```python
from build123d import *

# Parameters (mm, degrees)
CORTAR_EXTRUIR1_DEPTH      = 10
CORTAR_EXTRUIR1_DEPTH_BACK = 10
CROQUIS2_W                 = 11.9
CROQUIS2_H                 = 2.7
CORTAR_EXTRUIR2_DEPTH      = 10
CORTAR_EXTRUIR2_DEPTH_BACK = 10
CROQUIS4_W                 = 1
CROQUIS4_H                 = 10


with BuildPart() as part:
    # Croquis1 → Revoluci_n1 (revolve)
    with BuildSketch(Plane.XY, mode=Mode.PRIVATE) as revoluci_n1_sk:
        Polygon((-0.440734801, 5.95), (50.059265199, 5.95), (50.059265199, 4.95), (54.059265199, 4.1), (54.059265199, 0), (0, 0), (-0.440734801, 0), align=None)
    revolve(revoluci_n1_sk.sketch.rotate(Axis((54.059265199, 0, 0), (-1, 0, 0)), 90), axis=Axis((54.059265199, 0, 0), (-1, 0, 0)))

    # Croquis2 → Cortar-Extruir1 (cut, two sides: drawn at the far end of the back side and taken through both)
    with BuildSketch(Plane.XY.offset(-CORTAR_EXTRUIR1_DEPTH_BACK)):
        with Locations((5.509265199, 0)):
            Rectangle(CROQUIS2_W, CROQUIS2_H)
    extrude(amount=CORTAR_EXTRUIR1_DEPTH + CORTAR_EXTRUIR1_DEPTH_BACK, mode=Mode.SUBTRACT)

    # Croquis3 → Cortar-Extruir2 (cut, two sides: drawn at the far end of the back side and taken through both)
    with BuildSketch(Plane(origin=(0, 0, 0), x_dir=(1, 0, 0), z_dir=(0, 1, 0)).offset(-CORTAR_EXTRUIR2_DEPTH_BACK)):
        with BuildLine():
            ThreePointArc((3.359265199, 0), (4.859265199, -1.5), (6.359265199, 0))
            Line((6.359265199, 0), (3.359265199, 0))
        make_face()
        with BuildLine():
            Line((3.359265199, 0), (6.359265199, 0))
            ThreePointArc((6.359265199, 0), (4.859265199, 1.5), (3.359265199, 0))
        make_face()
    extrude(amount=CORTAR_EXTRUIR2_DEPTH + CORTAR_EXTRUIR2_DEPTH_BACK, mode=Mode.SUBTRACT)

    # Croquis4 → Revoluci_n2 (revolve)
    with BuildSketch(Plane(origin=(0, 0, 0), x_dir=(1, 0, 0), z_dir=(0, 1, 0))):
        with Locations((13.459265199, 5)):
            Rectangle(CROQUIS4_W, CROQUIS4_H)
    revolve(axis=Axis((0, 0, 0), (1, 0, 0)))


solid = part.part
```
Geometry check sheet. Reference: the model listing, model coordinates, mm. A direction names the side the tool comes from. Round coordinates to 2 decimals unless told otherwise and drop trailing zeros. Loops run counter-clockwise (first coordinate to the right, second up) from the corner with the lowest first, then second, coordinate; pieces in that order, holes last. Notation, with made-up numbers: (44.25, -29) - (55.25, -29) arc R33 ccw to (55.25, 9) - close; hole circle Ø5 at (57, -14). An arc over 180 degrees is marked (long way). Write each question's results on one line, items separated by ' | '. Start each with the question number.
Q1. Release check for a two-part mould opening along Y. For faces 1 (the flat face through (50.059, -4, 4)), 2 (the flat face through (7, 1.35, 0)), 3 (the cylindrical face through (32.262, -4.021, 4.385)) record: +Y half, -Y half, draft (parallel to the pull), parting line (faces both ways), or undercut.
Q2. Cross-section at B-B on y = 0. Enter the section's corners in (x, z), and give its area (3 significant figures).
Q3. Cross-section at A-A on z = 0. Enter the section's corners in (x, y).
Q4. Gauge pin test, flat ends, axial feed: P1, Ø4, axis at x = 4.86, z = 0, coming from the -Y side; P2, Ø5, axis at x = 27.5, z = 0, coming from the +Y side; P3, Ø3.5, axis at x = 8, z = 2, coming from the -Y side; P4, Ø10, axis at x = 18.5, z = 2, coming from the -Y side. Record the tip position at first contact, or that the pin passes through.
Q5. Thickness scan on line 1 (X direction, y = 3.3, z = 0); line 2 (X direction, y = 0, z = -3); line 3 (X direction, y = -5, z = 0.25). Record the ranges inside material, lowest first. Write a range as [from, to].
Q6. Cross-section at C-C on x = 28.5. Enter the section's corners in (y, z), and give its area (3 significant figures).
Q7. Access from +Z, -Z, +X, -X, +Y, -Y to the whole of each face (thin tool, end or side, straight path). Record for faces 4 (the flat face through (13.959, 0, 7)), 5 (the flat face through (7, -1.35, 0)), 6 (the flat face through (12.959, 0, 7)), 7 (the cylindrical face through (3.36, -3.68, -0.07)).
Q8. Cross-section at D-D on z = 6.5. Enter the section's corners in (x, y).
Answers below:
1) face 1: draft | face 2: undercut | face 3: parting line
2) outline: (11.46, -5.95) - (12.96, -5.95) - (12.96, -10) - (13.96, -10) - (13.96, -5.95) - (50.06, -5.95) - (50.06, -4.95) - (54.06, -4.1) - (54.06, 4.1) - (50.06, 4.95) - (50.06, 5.95) - (13.96, 5.95) - (13.96, 10) - (12.96, 10) - (12.96, 5.95) - (11.46, 5.95) - close | area: 504 mm²
3) outline: (-0.44, -5.95) - (3.36, -5.95) - (3.36, -1.35) - (-0.44, -1.35) - close; (-0.44, 1.35) - (3.36, 1.35) - (3.36, 5.95) - (-0.44, 5.95) - close; (6.36, -5.95) - (12.96, -5.95) - (12.96, -10) - (13.96, -10) - (13.96, -5.95) - (50.06, -5.95) - (50.06, -4.95) - (54.06, -4.1) - (54.06, 4.1) - (50.06, 4.95) - (50.06, 5.95) - (13.96, 5.95) - (13.96, 10) - (12.96, 10) - (12.96, 5.95) - (6.36, 5.95) - (6.36, 1.35) - (11.46, 1.35) - (11.46, -1.35) - (6.36, -1.35) - close
4) P1: stops at y = -5.95 | P2: stops at y = 5.95 | P3: stops at y = -5.94 | P4: stops at y = -10
5) line 1: x = [-0.44, 3.36], [6.36, 54.06] | line 2: x = [11.46, 54.06] | line 3: x = [-0.44, 3.38], [6.34, 50.06]
6) outline: circle Ø11.9 at (0, 0) | area: 111 mm²
7) face 4: +X | face 5: +Z, -Z, -X | face 6: -X | face 7: +Y, -Y
8) outline: (12.96, -7.6) - (13.96, -7.6) - (13.96, 7.6) - (12.96, 7.6) - close
